```python
from build123d import *

# Parameters (mm, degrees)
SALIENTE_EXTRUIR1_DEPTH = 2
CORTAR_EXTRUIR2_START   = -100
CORTAR_EXTRUIR2_DEPTH   = 100
CORTAR_EXTRUIR3_DEPTH   = 2
CROQUIS7_W              = 12
CROQUIS7_H              = 25
CORTAR_EXTRUIR4_DEPTH   = 2
CORTAR_EXTRUIR5_START   = -51.502837
CROQUIS9_W              = 2
CROQUIS9_H              = 6
CORTAR_EXTRUIR5_DEPTH   = 51.502837


with BuildPart() as part:
    # Croquis1 → Saliente-Extruir1 (new body)
    with BuildSketch(Plane.XY):
        Polygon((100, 100), (100, 42), (76, 42), (76, 0), (24, 0), (24, 42), (0, 42), (0, 100), align=None)
    extrude(amount=SALIENTE_EXTRUIR1_DEPTH)

    # Croquis4 → Cortar-Extruir2 (cut)
    with BuildSketch(Plane.ZY.offset(CORTAR_EXTRUIR2_START)):
        Polygon((2, 89.065555864), (2, 91.065555864), (2, 93.066666667), (2, 100), (0, 100), (0, 96.533333333), (0, 94.532222531), (0, 92.532222531), align=None)
    extrude(amount=CORTAR_EXTRUIR2_DEPTH, mode=Mode.SUBTRACT)

    # Croquis6 → Cortar-Extruir3 (cut)
    with BuildSketch(Plane(origin=(0, 0, 0), x_dir=(-1, 0, 0), z_dir=(0, 0, -1))):
        Polygon((-100, 92.532222531), (-99.5, 92.532222531), (-99.5, 42.5), (-75.502836605, 42.5), (-75.502836605, 0), (-76, 0), (-76, 42), (-100, 42), align=None)
    extrude(amount=-CORTAR_EXTRUIR3_DEPTH, mode=Mode.SUBTRACT)

    # Croquis7 → Cortar-Extruir4 (cut)
    with BuildSketch(Plane(origin=(0, 0, 0), x_dir=(-1, 0, 0), z_dir=(0, 0, -1))):
        with Locations((-49.75, 80.032222531)):
            Rectangle(CROQUIS7_W, CROQUIS7_H)
    extrude(amount=-CORTAR_EXTRUIR4_DEPTH, mode=Mode.SUBTRACT)

    # Croquis9 → Cortar-Extruir5 (cut)
    with BuildSketch(Plane(origin=(75.502836605, 0, 0), x_dir=(0, 0, -1), z_dir=(1, 0, 0)).offset(CORTAR_EXTRUIR5_START)):
        with Locations((-1, 3)):
            Rectangle(CROQUIS9_W, CROQUIS9_H)
    extrude(amount=CORTAR_EXTRUIR5_DEPTH, mode=Mode.SUBTRACT)


solid = part.part
```
Geometry: final body of the model. Coordinates: model frame, mm. A direction names the side the tool comes from. Coordinates: 2 decimals unless noted, no trailing zeros. Loops run counter-clockwise (first coordinate to the right, second up) from the corner with the lowest first, then second, coordinate; pieces in that order, holes last. Notation, with made-up numbers: (-10, 40) -> (44, 40) arc R12 cw to (44, 58) -> close; hole circle Ø7 at (81.5, 52.25). An arc over 180 degrees is marked (long way). Use a Markdown table: item, result. Add a question column.
(1) Line query: line 1 along X through (y, z) = (84.5, 0.75); line 2 along Y through (x, z) = (48, 1.3); line 3 along X through (y, z) = (14, 1.55). Output: solid intervals per line, ascending.
(2) Access query for faces 5 (the flat face through (43.75, 80, 1)), 6 (the flat face through (24, 24, 1)), 7 (the flat face through (0, 67, 1)), 8 (the flat face through (88, 42.5, 1)). Directions: +Z, -Z, +X, -X, +Y, -Y. A direction counts if a zero-diameter tool reaches every point of the face in a straight line with its end or side. Return the directions, or none.
(3) Section query C-C, the plane x = 36.5. Return loops of the section in (y, z), plus the area to 3 significant figures.
(4) Section query A-A, the plane y = 80. Return loops of the section in (x, z), plus the area to 3 significant figures.
(5) Section query D-D, the plane x = 85. Return loops of the section in (y, z).
(6) Section query B-B, the plane z = 1.15. Return loops of the section in (x, y).
(7) Mould query, pull axis X, two halves, no side actions, for faces 1 (the flat face through (55.75, 80, 1)), 2 (the flat face through (75.503, 25, 1)), 3 (the flat face through (50, 57, 2)), 4 (the flat face through (50, 67.532, 1)). Classes: pulls with the +X half, pulls with the -X half, needs draft (parallel to the pull), parting line crosses it, or undercut.
(8) Pin query (flat end, axial travel): pin 1 Ø0.6 at (y, z) = (31, 1) entering from +X. Return the tip coordinate at first contact, or that it passes through.
Answer:
| question | item | result |
|---|---|---|
| 1 | line 1 | x = 0 to 43.75, 55.75 to 99.5 |
| 1 | line 2 | y = 6 to 67.53 |
| 1 | line 3 | x = 24 to 75.5 |
| 2 | face 5 | +Z, -Z, +Y |
| 2 | face 6 | +Z, -Z, -X, -Y |
| 2 | face 7 | +Z, -Z, -X, +Y, -Y |
| 2 | face 8 | +Z, -Z, +X, -Y |
| 3 | outline | (6, 0) -> (92.53, 0) -> (89.07, 2) -> (6, 2) -> close |
| 3 | area | 170 mm^2 |
| 4 | outline | (0, 0) -> (43.75, 0) -> (43.75, 2) -> (0, 2) -> close; (55.75, 0) -> (99.5, 0) -> (99.5, 2) -> (55.75, 2) -> close |
| 4 | area | 175 mm^2 |
| 5 | outline | (42.5, 0) -> (92.53, 0) -> (89.07, 2) -> (42.5, 2) -> close |
| 6 | outline | (0, 42) -> (24, 42) -> (24, 6) -> (75.5, 6) -> (75.5, 42.5) -> (99.5, 42.5) -> (99.5, 90.54) -> (55.75, 90.54) -> (55.75, 67.53) -> (43.75, 67.53) -> (43.75, 90.54) -> (0, 90.54) -> close |
| 7 | face 1 | undercut |
| 7 | face 2 | pulls with the +X half |
| 7 | face 3 | needs draft |
| 7 | face 4 | undercut |
| 8 | pin 1 | stops at x = 75.5 |
